from build123d import *

# Parameters (mm, degrees)
BOSS_EXTRUDE1_DEPTH = 6.5
CUT_EXTRUDE1_DEPTH  = 9.5


with BuildPart() as part:
    # Sketch1 → Revolve1 (revolve)
    with BuildSketch(Plane(origin=(0, 158.016793392, -65.84033058), x_dir=(1, 0, 0), z_dir=(0, 0.923076923, -0.384615385))):
        Polygon((-20.075714319, 213.91124457), (-10.575714319, 213.91124457), (-10.575714319, 204.91124457), (-12.075714319, 204.91124457), (-12.075714319, 206.91124457), (-18.575714319, 206.91124457), (-18.575714319, 204.91124457), (-20.075714319, 204.91124457), align=None)
    revolve(axis=Axis((-11.075714319, 75.743237788, -263.296864029), (-1, 0, 0)))

    # Sketch2 → Boss-Extrude1 (add)
    with BuildSketch(Plane(origin=(-18.575714319, 0, 0), x_dir=(0, 0, -1), z_dir=(1, 0, 0))):
        with BuildLine():
            Line((263.396864029, 68.74395211), (263.396864029, 68.289102327))
            Line((263.396864029, 68.289102327), (262.496864029, 68.289102327))
            Line((262.496864029, 68.289102327), (262.496864029, 68.789102327))
            ThreePointArc((262.496864029, 68.789102327), (262.946136734, 68.752029711), (263.396864029, 68.74395211))
        make_face()
        with BuildLine():
            Line((261.65307078, 68.938978551), (261.539954239, 68.498418711))
            Line((261.539954239, 68.498418711), (260.668229394, 68.72223961))
            Line((260.668229394, 68.72223961), (260.792574337, 69.20653119))
            ThreePointArc((260.792574337, 69.20653119), (261.218512729, 69.058893701), (261.65307078, 68.938978551))
        make_face()
        with BuildLine():
            Line((260.012563106, 69.561541625), (259.793437552, 69.162953722))
            Line((259.793437552, 69.162953722), (259.00476154, 69.596532029))
            Line((259.00476154, 69.596532029), (259.245638377, 70.034685369))
            ThreePointArc((259.245638377, 70.034685369), (259.621479181, 69.785759612), (260.012563106, 69.561541625))
        make_face()
        with BuildLine():
            Line((258.578420138, 70.572523404), (258.267054035, 70.240952182))
            Line((258.267054035, 70.240952182), (257.610982271, 70.857044577))
            Line((257.610982271, 70.857044577), (257.953255824, 71.221528891))
            ThreePointArc((257.953255824, 71.221528891), (258.255383579, 70.886955787), (258.578420138, 70.572523404))
        make_face()
        with BuildLine():
            Line((257.440754352, 71.908400183), (257.056711979, 71.664679482))
            Line((257.056711979, 71.664679482), (256.574467864, 72.424574615))
            Line((256.574467864, 72.424574615), (256.996631826, 72.692488013))
            ThreePointArc((256.996631826, 72.692488013), (257.206062735, 72.293290021), (257.440754352, 71.908400183))
        make_face()
        with BuildLine():
            Line((256.671049475, 73.485233913), (256.238461626, 73.3446776))
            Line((256.238461626, 73.3446776), (255.960346331, 74.200628465))
            Line((255.960346331, 74.200628465), (256.435874589, 74.355136962))
            ThreePointArc((256.435874589, 74.355136962), (256.539449337, 73.91639716), (256.671049475, 73.485233913))
        make_face()
        with BuildLine():
            Line((256.317668895, 75.203946331), (255.863716654, 75.175386077))
            Line((255.863716654, 75.175386077), (255.807205187, 76.073610132))
            Line((255.807205187, 76.073610132), (256.306218551, 76.105005392))
            ThreePointArc((256.306218551, 76.105005392), (256.297429156, 75.654291415), (256.317668895, 75.203946331))
        make_face()
        with BuildLine():
            Line((256.402816812, 76.956544414), (255.95602367, 77.041774764))
            Line((255.95602367, 77.041774764), (256.124666853, 77.92583329))
            Line((256.124666853, 77.92583329), (256.615810478, 77.832142633))
            ThreePointArc((256.615810478, 77.832142633), (256.49520921, 77.397774498), (256.402816812, 76.956544414))
        make_face()
        with BuildLine():
            Line((256.921143071, 78.63290598), (256.509582683, 78.826571598))
            Line((256.509582683, 78.826571598), (256.892784045, 79.640915945))
            Line((256.892784045, 79.640915945), (257.345197571, 79.428026299))
            ThreePointArc((257.345197571, 79.428026299), (257.120362252, 79.037296954), (256.921143071, 78.63290598))
        make_face()
        with BuildLine():
            Line((257.840079325, 80.127699066), (257.489611545, 80.417631229))
            Line((257.489611545, 80.417631229), (258.063293135, 81.111093147))
            Line((258.063293135, 81.111093147), (258.448549757, 80.792381152))
            ThreePointArc((258.448549757, 80.792381152), (258.133607615, 80.469841558), (257.840079325, 80.127699066))
        make_face()
        with BuildLine():
            Line((259.101885432, 81.347000324), (258.834531438, 81.714981528))
            Line((258.834531438, 81.714981528), (259.562646733, 82.243988255))
            Line((259.562646733, 82.243988255), (259.856539359, 81.839479758))
            ThreePointArc((259.856539359, 81.839479758), (259.471279368, 81.605396264), (259.101885432, 81.347000324))
        make_face()
        with BuildLine():
            Line((260.627277471, 82.214196574), (260.459836099, 82.637105206))
            Line((260.459836099, 82.637105206), (261.296634936, 82.968417303))
            Line((261.296634936, 82.968417303), (261.480697212, 82.50352906))
            ThreePointArc((261.480697212, 82.50352906), (261.049326675, 82.372609993), (260.627277471, 82.214196574))
        make_face()
        with BuildLine():
            Line((262.320409452, 82.674798684), (262.263401658, 83.12606184))
            Line((262.263401658, 83.12606184), (263.15630489, 83.23886175))
            Line((263.15630489, 83.23886175), (263.218971506, 82.7428044))
            ThreePointArc((263.218971506, 82.7428044), (262.76859502, 82.723275886), (262.320409452, 82.674798684))
        make_face()
        with BuildLine():
            Line((264.074895666, 82.699865331), (264.13190346, 83.151128487))
            Line((264.13190346, 83.151128487), (265.024806691, 83.038328577))
            Line((265.024806691, 83.038328577), (264.962140074, 82.542271226))
            ThreePointArc((264.962140074, 82.542271226), (264.52105645, 82.635360314), (264.074895666, 82.699865331))
        make_face()
        with BuildLine():
            Line((265.78049529, 82.287821484), (265.947936663, 82.710730117))
            Line((265.947936663, 82.710730117), (266.7847355, 82.379418019))
            Line((266.7847355, 82.379418019), (266.600673224, 81.914529776))
            ThreePointArc((266.600673224, 81.914529776), (266.196597367, 82.114387336), (265.78049529, 82.287821484))
        make_face()
        with BuildLine():
            Line((267.330039228, 81.464557375), (267.597393222, 81.832538579))
            Line((267.597393222, 81.832538579), (268.325508517, 81.303531852))
            Line((268.325508517, 81.303531852), (268.031615891, 80.899023354))
            ThreePointArc((268.031615891, 80.899023354), (267.689937374, 81.193091601), (267.330039228, 81.464557375))
        make_face()
        with BuildLine():
            Line((268.626163935, 80.281801714), (268.976631716, 80.571733877))
            Line((268.976631716, 80.571733877), (269.550313307, 79.878271959))
            Line((269.550313307, 79.878271959), (269.165056685, 79.559559964))
            ThreePointArc((269.165056685, 79.559559964), (268.907244427, 79.929361507), (268.626163935, 80.281801714))
        make_face()
        with BuildLine():
            Line((269.587429129, 78.81387139), (269.998989517, 79.007537008))
            Line((269.998989517, 79.007537008), (270.38219088, 78.193192661))
            Line((270.38219088, 78.193192661), (269.929777353, 77.980303015))
            ThreePointArc((269.929777353, 77.980303015), (269.772030645, 78.402601865), (269.587429129, 78.81387139))
        make_face()
        with BuildLine():
            Line((270.153434983, 77.153001864), (270.600228126, 77.238232214))
            Line((270.600228126, 77.238232214), (270.768871309, 76.354173689))
            Line((270.768871309, 76.354173689), (270.277727683, 76.260483031))
            ThreePointArc((270.277727683, 76.260483031), (270.229958331, 76.708744597), (270.153434983, 77.153001864))
        make_face()
        with BuildLine():
            Line((270.288617268, 75.403551676), (270.742569508, 75.374991422))
            Line((270.742569508, 75.374991422), (270.68605804, 74.476767367))
            Line((270.68605804, 74.476767367), (270.187044676, 74.508162626))
            ThreePointArc((270.187044676, 74.508162626), (270.252254204, 74.954220986), (270.288617268, 75.403551676))
        make_face()
        with BuildLine():
            Line((269.984481982, 73.675445216), (270.417069832, 73.534888904))
            Line((270.417069832, 73.534888904), (270.138954537, 72.678938039))
            Line((270.138954537, 72.678938039), (269.663426278, 72.833446536))
            ThreePointArc((269.663426278, 72.833446536), (269.837517332, 73.249274201), (269.984481982, 73.675445216))
        make_face()
        with BuildLine():
            Line((269.260139065, 72.077265768), (269.644181438, 71.833545067))
            Line((269.644181438, 71.833545067), (269.161937323, 71.073649934))
            Line((269.161937323, 71.073649934), (268.73977336, 71.341563332))
            ThreePointArc((268.73977336, 71.341563332), (269.011807158, 71.701032322), (269.260139065, 72.077265768))
        make_face()
        with BuildLine():
            Line((268.161101646, 70.709432825), (268.472467748, 70.377861603))
            Line((268.472467748, 70.377861603), (267.816395984, 69.761769208))
            Line((267.816395984, 69.761769208), (267.474122431, 70.126253522))
            ThreePointArc((267.474122431, 70.126253522), (267.82700609, 70.406777078), (268.161101646, 70.709432825))
        make_face()
        with BuildLine():
            Line((266.756426289, 69.65789236), (266.975551842, 69.259304457))
            Line((266.975551842, 69.259304457), (266.18687583, 68.825726151))
            Line((266.18687583, 68.825726151), (265.945998993, 69.263879491))
            ThreePointArc((265.945998993, 69.263879491), (266.357559535, 69.447831286), (266.756426289, 69.65789236))
        make_face()
        with BuildLine():
            Line((265.134373911, 68.988716529), (265.247490452, 68.548156689))
            Line((265.247490452, 68.548156689), (264.375765607, 68.32433579))
            Line((264.375765607, 68.32433579), (264.251420663, 68.808627371))
            ThreePointArc((264.251420663, 68.808627371), (264.695798225, 68.884449038), (265.134373911, 68.988716529))
        make_face()
    extrude(amount=BOSS_EXTRUDE1_DEPTH)

    # Sketch3 → Cut-Extrude1 (cut)
    with BuildSketch(Plane(origin=(-10.575714319, 0, 0), x_dir=(0, 0, -1), z_dir=(1, 0, 0))):
        with BuildLine():
            Line((264.364668647, 74.465986264), (264.364668647, 76.963985463))
            ThreePointArc((264.364668647, 76.963985463), (261.764668647, 75.714985864), (264.364668647, 74.465986264))
        make_face()
    extrude(amount=-CUT_EXTRUDE1_DEPTH, mode=Mode.SUBTRACT)


solid = part.part
The listing builds one solid part. Answer for the finished solid, in the listing's coordinates (mm). A direction names the side the tool comes from. Coordinates: 2 decimals unless noted, no trailing zeros. Write each loop counter-clockwise with the first axis right and the second up, starting at its lowest first coordinate (ties: lowest second). Pieces come first, ordered by that corner, then holes. Notation, with made-up numbers: M 29.5,23 L 47.5,23 A10 ccw 47.5,34 Z; hole C -38.75,-32 d5. An arc over 180 degrees is marked long. Use one line per item in the form item = value.
Item 1: Find the intervals of material crossed by probe 1 along X at (y, z) = (82, -258.5); probe 2 along Y at (x, z) = (-14.5, -263.5); probe 3 along Z at (x, y) = (-10.75, 75.75), in increasing order.
Model answer:
probe_1 = -20.08 to -18.58, -12.08 to -10.58
probe_2 = 68.75 to 74.12, 77.31 to 82.74
probe_3 = -272.3 to -264.36, -261.77 to -254.3
Item 2: Find section A-A, the plane x = -11.25. Give the vertices of the cut face in (y, z), plus the area to 3 significant figures.
Model answer:
outline = C 75.74,-263.3 d18; hole M 74.47,-264.36 L 76.96,-264.36 A1.6 ccw long Z
area = 247 mm2
Item 3: For faces 1 (the face through (-15.37, 68.85, -262.08)), 2 (the face through (-15.37, 68.44, -264.82)), 3 (the face through (-15.37, 68.61, -261.11)), 4 (the face through (-15.37, 79.23, -256.7)), 5 (the face through (-15.371, 83.096, -264.572)), determine the directions among +Z, -Z, +X, -X, +Y, -Y from which every point of the face is accessible in a straight line to the end or side of a thin tool.
Model answer:
face_1 = -Y
face_2 = -Z, -Y
face_3 = +Z, -Y
face_4 = +Z, +Y
face_5 = -Z, +Y
Item 4: The mould has two halves that part along Z. Classify faces 6 (the face through (-15.37, 73.77, -256.1)), 7 (the face through (-15.371, 69.116, -265.55)), 8 (the face through (-15.37, 73.11, -270.28)), 9 (the face through (-20.076, 77, -262)): released by +Z, released by -Z, zero draft, split by the parting line, or undercut.
Model answer:
face_6 = released by +Z
face_7 = undercut
face_8 = released by -Z
face_9 = zero draft
Item 5: Given P1, Ø1, axis at x = -17.5, y = 72, coming from the +Z side; P2, Ø5, axis at x = -12.5, y = 69.5, coming from the +Z side; P3, Ø3, axis at x = -18.5, y = 69, coming from the -Z side, each flat-ended and moving along its own axis, determine where each tip first touches the part or whether it passes through.
Model answer:
P1 = -256.57
P2 = -255.13
P3 = -270.61
